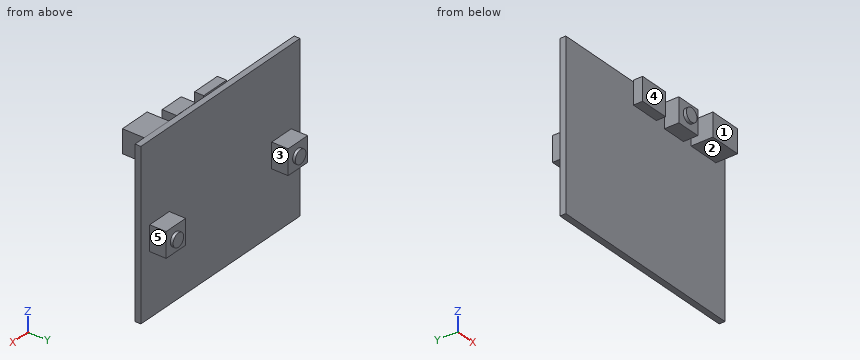
from build123d import *

# Parameters (mm, degrees)
ESQUISSE1_W        = 51.8
ESQUISSE1_H        = 42
BOSS_EXTRU_1_DEPTH = 1.5
ESQUISSE2_W        = 6.35
ESQUISSE2_H        = 6.35
BOSS_EXTRU_2_DEPTH = 4.17
ESQUISSE3_R        = 1.72
BOSS_EXTRU_3_DEPTH = 0.7
ESQUISSE7_W        = 6.16
ESQUISSE7_H        = 6.16
BOSS_EXTRU_4_DEPTH = 3.66
ESQUISSE5_W        = 7.44
ESQUISSE5_H        = 5.9
BOSS_EXTRU_5_DEPTH = 2.34
ESQUISSE6_W        = 8.04
ESQUISSE6_H        = 5.92
BOSS_EXTRU_6_DEPTH = 5.55
ESQUISSE8_R        = 1.72
BOSS_EXTRU_7_DEPTH = 0.8


with BuildPart() as part:
    # Esquisse1 → Boss.-Extru.1 (new body)
    with BuildSketch(Plane(origin=(0, 0, 0), x_dir=(1, 0, 0), z_dir=(0, 1, 0))):
        with Locations((25.9, 21)):
            Rectangle(ESQUISSE1_W, ESQUISSE1_H)
    extrude(amount=-BOSS_EXTRU_1_DEPTH)

    # Esquisse2 → Boss.-Extru.2 (add)
    with BuildSketch(Plane(origin=(0, 0, 0), x_dir=(1, 0, 0), z_dir=(0, 1, 0))):
        with Locations((45.745, 23.125)):
            Rectangle(ESQUISSE2_W, ESQUISSE2_H)
        with Locations((6.055, 23.125)):
            Rectangle(ESQUISSE2_W, ESQUISSE2_H)
    extrude(amount=BOSS_EXTRU_2_DEPTH)

    # Esquisse3 → Boss.-Extru.3 (add)
    with BuildSketch(Plane(origin=(0, 4.17, 0), x_dir=(1, 0, 0), z_dir=(0, 1, 0))):
        with Locations((6.030530149, 23.148945457)):
            Circle(ESQUISSE3_R)
        with Locations((45.817014074, 23.217873135)):
            Circle(ESQUISSE3_R)
    extrude(amount=BOSS_EXTRU_3_DEPTH)

    # Esquisse7 → Boss.-Extru.4 (add)
    with BuildSketch(Plane.XZ.offset(1.5)):
        with Locations((35.174690325, -3.02873507)):
            Rectangle(ESQUISSE7_W, ESQUISSE7_H)
    extrude(amount=BOSS_EXTRU_4_DEPTH)

    # Esquisse5 → Boss.-Extru.5 (add)
    with BuildSketch(Plane.XZ.offset(1.5)):
        with Locations((25.72, -2.536674281)):
            Rectangle(ESQUISSE5_W, ESQUISSE5_H)
    extrude(amount=BOSS_EXTRU_5_DEPTH)

    # Esquisse6 → Boss.-Extru.6 (add)
    with BuildSketch(Plane.XZ.offset(1.5)):
        with Locations((44.78, -2.971238989)):
            Rectangle(ESQUISSE6_W, ESQUISSE6_H)
    extrude(amount=BOSS_EXTRU_6_DEPTH)

    # Esquisse8 → Boss.-Extru.7 (add)
    with BuildSketch(Plane.XZ.offset(5.16)):
        with Locations((35.263038033, -2.994330068)):
            Circle(ESQUISSE8_R)
    extrude(amount=BOSS_EXTRU_7_DEPTH)


solid = part.part
CAD build for the part. Positions are in the model's coordinates, mm. Face numbers are marked on the shaded views. A direction names the side the tool comes from. Round coordinates to 2 decimals unless told otherwise and drop trailing zeros. Write each loop counter-clockwise with the first axis right and the second up, starting at its lowest first coordinate (ties: lowest second). Pieces come first, ordered by that corner, then holes.
(1) Drop flat-ended pins along their axis: P1, Ø3, axis at y = 2.5, z = -21.5, coming from the +X side; P2, Ø10, axis at x = 5, z = -6.5, coming from the +Y side; P3, Ø2, axis at x = 46, y = 1.5, coming from the -Z side. Give the stop position or say it passes through.
(2) Slice it at A-A, the plane y = 0.75. Write the cut outline in (x, z), and give its area (3 significant figures).
(3) 3-axis set-ups, long thin cutter, end or side, ignore diameter. For the marked faces 1 and 2: which of +Z, -Z, +X, -X, +Y, -Y reach the whole face in a straight line?
(4) Probe line 1 along X through (y, z) = (-2.25, -4.5); line 2 along Y through (x, z) = (8.5, -30); line 3 along Z through (x, y) = (36.5, -3.5). List the from-to ranges inside material, lowest first.
(5) Slice it at B-B, the plane x = 24.5. Write the cut outline in (y, z), and give its area (3 significant figures).
(6) Slice it at C-C, the plane z = -33. Write the cut outline in (x, y), and give its area (3 significant figures).
(7) Slice it at D-D, the plane x = 6. Write the cut outline in (y, z), and give its area (3 significant figures).
(8) Mould opens along X. For the marked faces 3, 4 and 5 say: pulls with the +X half, pulls with the -X half, needs draft (parallel to the pull), parting line crosses it, or undercut.
From the geometry:
1. P1: stops at x = 48.92
1. P2: stops at y = 0
1. P3: stops at z = -26.3
2. outline: (2.88, -26.3) - (9.23, -26.3) - (9.23, -19.95) - (2.88, -19.95) - close; (42.57, -26.3) - (48.92, -26.3) - (48.92, -19.95) - (42.57, -19.95) - close
2. area: 80.6 mm2
3. face 1: +Z, -Z, +X, -X, -Y
3. face 2: -Z, +X, -Y
4. line 1: x = 22 to 29.44, 32.09 to 38.25, 40.76 to 48.8
4. line 2: y = -1.5 to 0
4. line 3: z = -6.11 to 0.05
5. outline: (-3.84, -5.49) - (-1.5, -5.49) - (-1.5, -42) - (0, -42) - (0, 0) - (-1.5, 0) - (-1.5, 0.41) - (-3.84, 0.41) - close
5. area: 76.8 mm2
6. outline: (0, -1.5) - (51.8, -1.5) - (51.8, 0) - (0, 0) - close
6. area: 77.7 mm2
7. outline: (-1.5, -42) - (0, -42) - (0, -26.3) - (4.17, -26.3) - (4.17, -24.87) - (4.87, -24.87) - (4.87, -21.43) - (4.17, -21.43) - (4.17, -19.95) - (0, -19.95) - (0, 0) - (-1.5, 0) - close
7. area: 91.9 mm2
8. face 3: undercut
8. face 4: needs draft
8. face 5: pulls with the +X half
